CAD build for the part. Positions are in the model's coordinates, mm. Coordinates: 2 decimals unless noted, no trailing zeros. Order: outer loops, then holes, each group sorted by start corner. A loop starts at its lowest first (then second) coordinate and runs counter-clockwise, first axis right, second up. Notation, with made-up numbers: (49.25, 88.5) - (61.25, 88.5) arc R9 ccw to (61.25, 92.5) - close; hole circle Ø2 at (-33.75, 28). An arc over 180 degrees is marked (long way). Use one line per item in the form item = value.
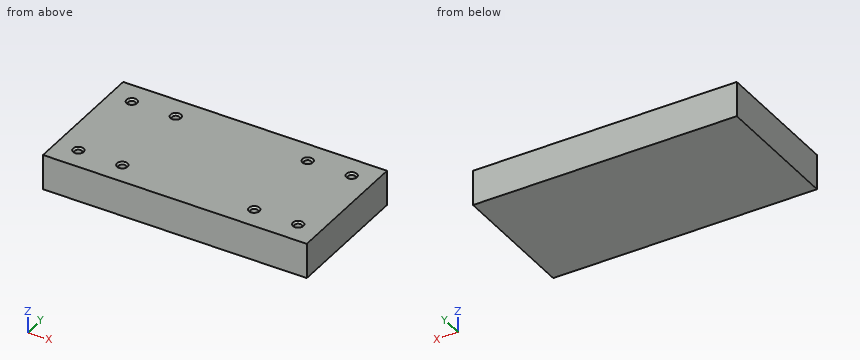
Autodesk Inventor part; units mm, degrees
ref_plane "YZ Plane" through (0, 0, 0) normal (1, 0, 0) x (0, 1, 0)
ref_plane "XZ Plane" through (0, 0, 0) normal (0, 1, 0) x (-1, 0, 0)
ref_plane "XY Plane" through (0, 0, 0) normal (0, 0, 1) x (1, 0, 0)
sketch "Esboço1" plane through (0, 0, 0) normal (0, 0, 1) x (1, 0, 0)
  line L0 (-300, -150) -> (300, -150)
  line L1 (300, -150) -> (300, 150)
  line L2 (300, 150) -> (-300, 150)
  line L3 (-300, 150) -> (-300, -150)
  line L4 (-300, -150) -> (300, 150) construction
  line L5 (300, -150) -> (-300, 150) construction
  point P0 (0, 0)
  dimension "d0" = 600
  dimension "d1" = 300
extrude "Extrusão1" add sketch "Esboço1" along normal blind 80
sketch "Esboço2" plane through (0, 0, 80) normal (0, 0, 1) x (1, 0, 0)
  line L0 (-250, -100) -> (250, -100)
  line L1 (250, -100) -> (250, 100)
  line L2 (250, 100) -> (-250, 100)
  line L3 (-250, 100) -> (-250, -100)
  line L4 (-250, -100) -> (250, 100) construction
  line L5 (250, -100) -> (-250, 100) construction
  line L6 (-150, -100) -> (150, -100)
  line L7 (150, -100) -> (150, 100)
  line L8 (150, 100) -> (-150, 100)
  line L9 (-150, 100) -> (-150, -100)
  line L10 (-150, -100) -> (150, 100) construction
  line L11 (150, -100) -> (-150, 100) construction
  circle A0 centre (-250, 100) radius 8
  circle A1 centre (-150, 100) radius 8
  circle A2 centre (150, 100) radius 8
  circle A3 centre (250, 100) radius 8
  circle A4 centre (250, -100) radius 8
  circle A5 centre (150, -100) radius 8
  circle A6 centre (-150, -100) radius 8
  circle A7 centre (-250, -100) radius 8
  point P0 (0, 0)
  dimension "d4" = 500
  dimension "d5" = 200
  dimension "d6" = 300
  dimension "d7" = 16
  dimension "d8" = 16
  dimension "d9" = 16
  dimension "d10" = 16
  dimension "d11" = 16
  dimension "d12" = 16
  dimension "d13" = 16
  dimension "d14" = 16
extrude "Extrusão2" cut sketch "Esboço2" against normal blind 40 contours L3 A7 L0 | L0 A7 L3 | A6 L9 L0 | L0 A6 | A0 L2 L3 | L3 L2 A0 | L9 A6 L0 | A1 L2 L9 | L9 L2 A1 | A5 L7 L0 | L0 A5 | A1 L2 | L7 A5 L0 | A2 L2 | L2 L7 A2 | L7 L2 A2 | A4 L1 L0 | L0 L1 A4 | A3 L1 L2 | L2 L1 A3
chamfer "Chanfro1" distance 4 angle 45 8 edges at (-258, 100, 80) (-158, 100, 80) (-258, -100, 80) (-158, -100, 80) (142, 100, 80) (142, -100, 80) (242, 100, 80) (242, -100, 80)
properties part number "suporte topo"
Item 1: Drill centre lines: line 1 (X direction, y = -100, z = 50); line 2 (Y direction, x = 150, z = 57). Where is each one in solid material? Low to high. Write a range as [from, to].
Derived:
line_1 = [-300, -258], [-242, -158], [-142, 142], [158, 242], [258, 300]
line_2 = [-150, -108], [-92, 92], [108, 150]
Item 2: Cut at A-A, the plane y = 100. Write the cut outline in (x, z), plus the area to 3 significant figures.
Derived:
outline = (-300, 0) - (300, 0) - (300, 80) - (262, 80) - (258, 76) - (258, 40) - (242, 40) - (242, 76) - (238, 80) - (162, 80) - (158, 76) - (158, 40) - (142, 40) - (142, 76) - (138, 80) - (-138, 80) - (-142, 76) - (-142, 40) - (-158, 40) - (-158, 76) - (-162, 80) - (-238, 80) - (-242, 76) - (-242, 40) - (-258, 40) - (-258, 76) - (-262, 80) - (-300, 80) - close
area = 45,400 mm²
Item 3: Cut at B-B, the plane x = 150. Write the cut outline in (y, z), plus the area to 3 significant figures.
Derived:
outline = (-150, 0) - (150, 0) - (150, 80) - (112, 80) - (108, 76) - (108, 40) - (92, 40) - (92, 76) - (88, 80) - (-88, 80) - (-92, 76) - (-92, 40) - (-108, 40) - (-108, 76) - (-112, 80) - (-150, 80) - close
area = 22,700 mm²
Item 4: Drop flat-ended pins along their axis: pin 1 (13 mm diameter, centred on x = 152, y = -101.5, fed in from +Z); pin 2 (13 mm diameter, centred on x = 250, y = -100, fed in from +Z); pin 3 (21 mm diameter, centred on x = -150, y = 100, fed in from +Z). Give the stop position or say it passes through.
Derived:
pin_1 = 77
pin_2 = 40
pin_3 = 78.5
